The drawing under review shows one solid part. Ordinate dimensions are in mm from its lowest x, y, z. A direction names the side the tool comes from. Coordinates: 2 decimals unless noted, no trailing zeros. Loops run counter-clockwise (first coordinate to the right, second up) from the corner with the lowest first, then second, coordinate; pieces in that order, holes last. Notation, with made-up numbers: (67, 59.5) -> (83, 59.5) arc R15 ccw to (83, 75.5) -> close; hole circle Ø1 at (22, 46). An arc over 180 degrees is marked (long way). Use a Markdown table: item, result.
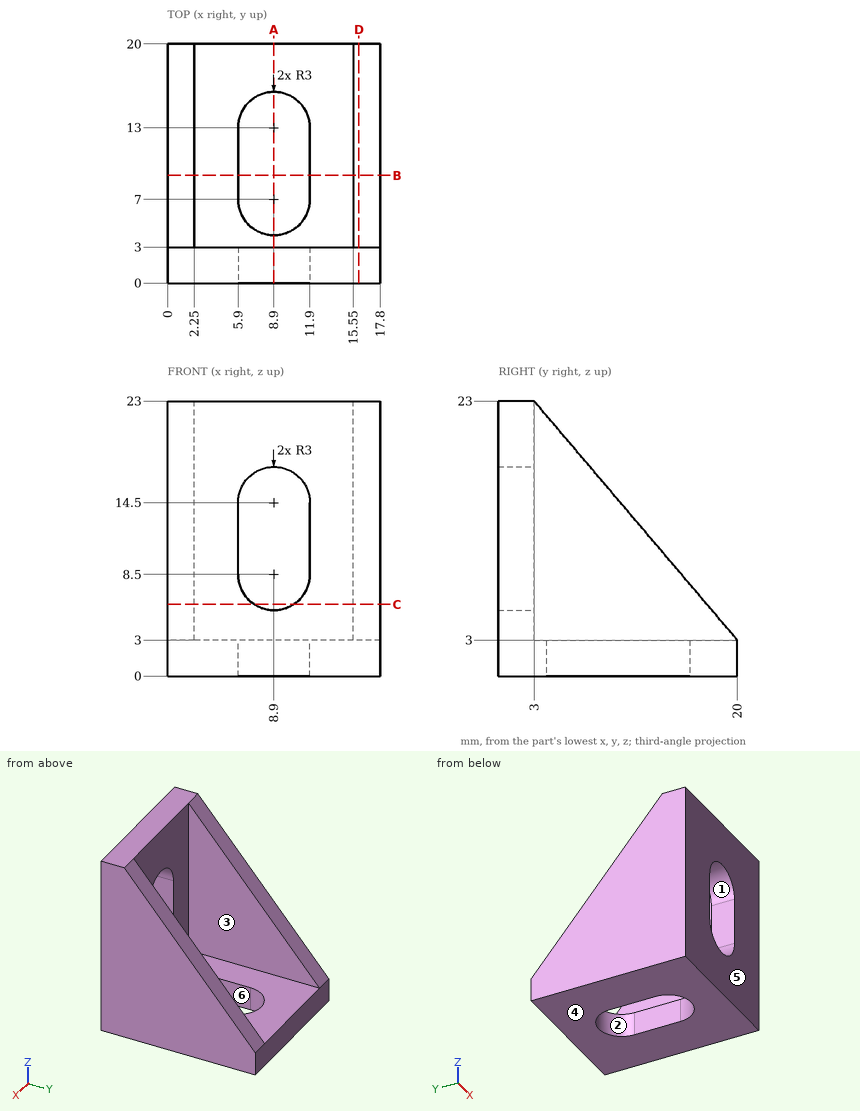
(1) For line 1 along X through (y, z) = (11.25, 1); line 2 along X through (y, z) = (6, 11); line 3 along Y through (x, z) = (14.5, 13.25), list the stretches that pass through material, from the lowest coordinate up.
Found:
| item | result |
|---|---|
| line 1 | x = 0 to 5.9, 11.9 to 17.8 |
| line 2 | x = 0 to 2.25, 15.55 to 17.8 |
| line 3 | y = 0 to 3 |
(2) Mouldability with a two-part tool opening along Y and no side actions: class the marked faces 4, 5 and 6 as pulls with the +Y half, pulls with the -Y half, needs draft (parallel to the pull), parting line crosses it, or undercut.
Found:
| item | result |
|---|---|
| face 4 | needs draft |
| face 5 | pulls with the -Y half |
| face 6 | undercut |
(3) Take a section at B-B on y = 9. Write out the cut boundary in (x, z), plus the area to 3 significant figures.
Found:
| item | result |
|---|---|
| outline | (0, 0) -> (5.9, 0) -> (5.9, 3) -> (2.25, 3) -> (2.25, 15.94) -> (0, 15.94) -> close; (11.9, 0) -> (17.8, 0) -> (17.8, 15.94) -> (15.55, 15.94) -> (15.55, 3) -> (11.9, 3) -> close |
| area | 93.6 mm^2 |
(4) Take a section at A-A on x = 8.9. Write out the cut boundary in (y, z), plus the area to 3 significant figures.
Found:
| item | result |
|---|---|
| outline | (0, 0) -> (4, 0) -> (4, 3) -> (3, 3) -> (3, 5.5) -> (0, 5.5) -> close; (0, 17.5) -> (3, 17.5) -> (3, 23) -> (0, 23) -> close; (16, 0) -> (20, 0) -> (20, 3) -> (16, 3) -> close |
| area | 48.0 mm^2 |
(5) Take a section at D-D on x = 16. Write out the cut boundary in (y, z).
Found:
| item | result |
|---|---|
| outline | (0, 0) -> (20, 0) -> (20, 3) -> (3, 23) -> (0, 23) -> close |
(6) For pin 1 Ø1.5 at (x, z) = (12, 9.5) entering from +Y; pin 2 Ø0.9 at (y, z) = (1, 12.5) entering from -X, all flat-tipped, find the tip position at first contact; note any pin that passes through.
Found:
| item | result |
|---|---|
| pin 1 | stops at y = 3 |
| pin 2 | stops at x = 0 |
(7) Take a section at C-C on z = 6. Write out the cut boundary in (x, y).
Found:
| item | result |
|---|---|
| outline | (0, 0) -> (7.24, 0) -> (7.24, 3) -> (2.25, 3) -> (2.25, 17.45) -> (0, 17.45) -> close; (10.56, 0) -> (17.8, 0) -> (17.8, 17.45) -> (15.55, 17.45) -> (15.55, 3) -> (10.56, 3) -> close |
(8) For the marked faces 1, 2 and 3, list the 3-axis set-ups (+Z, -Z, +X, -X, +Y, -Y) from which the entire face can be reached by the end or side of a thin tool; tool diameter is ignored.
Found:
| item | result |
|---|---|
| face 1 | +Y, -Y |
| face 2 | +Z, -Z |
| face 3 | +Z, +Y |
